Here's how the part is built. I have some questions about the finished solid (model axes, mm). Face numbers are marked on the shaded views. Coordinates: 2 decimals unless noted, no trailing zeros. Loops run counter-clockwise (first coordinate to the right, second up) from the corner with the lowest first, then second, coordinate; pieces in that order, holes last. Notation, with made-up numbers: (65.25, 73) -> (85.25, 73) arc R12 ccw to (85.25, 86) -> close; hole circle Ø3 at (-8.5, 76.5). An arc over 180 degrees is marked (long way). Use CSV: the item, a comma, the result in double quotes. Start each with the question number.
Autodesk Inventor part; units mm, degrees
ref_plane "YZ Plane" through (0, 0, 0) normal (1, 0, 0) x (0, 1, 0)
ref_plane "XZ Plane" through (0, 0, 0) normal (0, 1, 0) x (-1, 0, 0)
ref_plane "XY Plane" through (0, 0, 0) normal (0, 0, 1) x (1, 0, 0)
sketch "Sketch1" plane through (0, 0, 0) normal (0, 1, 0) x (-1, 0, 0)
  line L0 (-5, -2.5) -> (5, -2.5)
  line L1 (5, 2.5) -> (5, 2.5)
  line L2 (5, 2.5) -> (-5, 2.5)
  line L3 (-5, 2.5) -> (-5, 2.5)
  line L4 (-5, -2.5) -> (5, 2.5) construction
  line L5 (5, -2.5) -> (-5, 2.5) construction
  circle A0 centre (3, 0) radius 1
  circle A1 centre (-3, 0) radius 1
  line L6 (5, 2.5) -> (5, -2.5)
  line L7 (-5, 2.5) -> (-5, -2.5)
  point P0 (0, 0)
  dimension "d1" = 10
  dimension "d3" = 2
  dimension "d4" = 2
  dimension "d5" = 2
  dimension "d6" = 2
  dimension "d7" = 2.5
  dimension "d8" = 2.5
  dimension "d12" = 5
extrude "Extrusion1" add sketch "Sketch1" along normal blind 5
properties part number "link"
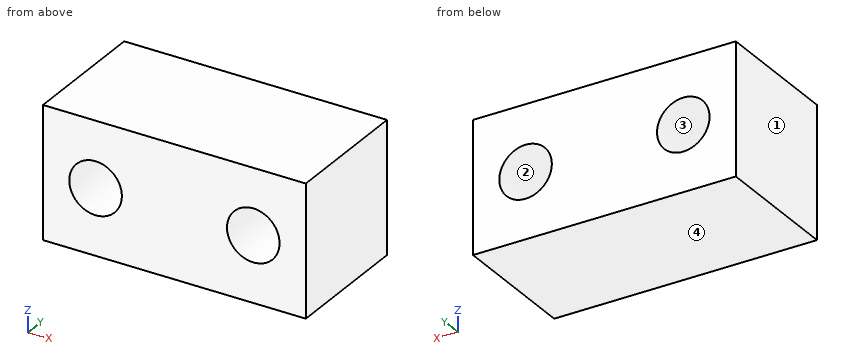
1) For P1, Ø1.6, axis at x = -3, z = 0, coming from the -Y side, with a flat end and sliding along its axis, tell me the tip position at first contact or that it passes through.
2) I want a section at A-A, the plane z = 0. Please give me the cut outline in (x, y), plus the area to 3 significant figures.
3) Please list where these lines run through material, in increasing order: L1, parallel to Z at x = -3, y = 3.2; L2, parallel to X at y = 4.5, z = 0.3; L3, parallel to X at y = 4.5, z = 0.85. Write a range as [from, to].
4) Thinking about a two-plate mould opening in Z: for the marked faces 1, 2, 3 and 4, which applies, pulls with the +Z half, pulls with the -Z half, needs draft (parallel to the pull), parting line crosses it, or undercut?
5) I want a section at C-C, the plane y = 2.55. Please give me the cut outline in (x, z), plus the area to 3 significant figures.
6) I want a section at B-B, the plane x = 3. Please give me the cut outline in (y, z), plus the area to 3 significant figures.
Return value:
1,P1,"passes through"
2,outline,"(-5, 0) -> (-4, 0) -> (-4, 5) -> (-5, 5) -> close; (-2, 0) -> (2, 0) -> (2, 5) -> (-2, 5) -> close; (4, 0) -> (5, 0) -> (5, 5) -> (4, 5) -> close"
2,area,"30.0 mm²"
3,L1,"z = [-2.5, -1], [1, 2.5]"
3,L2,"x = [-5, -3.95], [-2.05, 2.05], [3.95, 5]"
3,L3,"x = [-5, -3.53], [-2.47, 2.47], [3.53, 5]"
4,face 1,"needs draft"
4,face 2,"undercut"
4,face 3,"undercut"
4,face 4,"pulls with the -Z half"
5,outline,"(-5, -2.5) -> (5, -2.5) -> (5, 2.5) -> (-5, 2.5) -> close; hole circle Ø2 at (-3, 0); hole circle Ø2 at (3, 0)"
5,area,"43.7 mm²"
6,outline,"(0, -2.5) -> (5, -2.5) -> (5, -1) -> (0, -1) -> close; (0, 1) -> (5, 1) -> (5, 2.5) -> (0, 2.5) -> close"
6,area,"15.0 mm²"
